Check sheet for the drawn part. Datum: minimum x, y, z corner. Units: mm. A direction names the side the tool comes from. Coordinates: 2 decimals unless noted, no trailing zeros. Write each loop counter-clockwise with the first axis right and the second up, starting at its lowest first coordinate (ties: lowest second). Pieces come first, ordered by that corner, then holes. Notation, with made-up numbers: M 76,31 L 108,31 A15 ccw 108,35 Z; hole C 86,13.5 d8. An arc over 180 degrees is marked long. Write item = value, one per line. Start each with the question number.
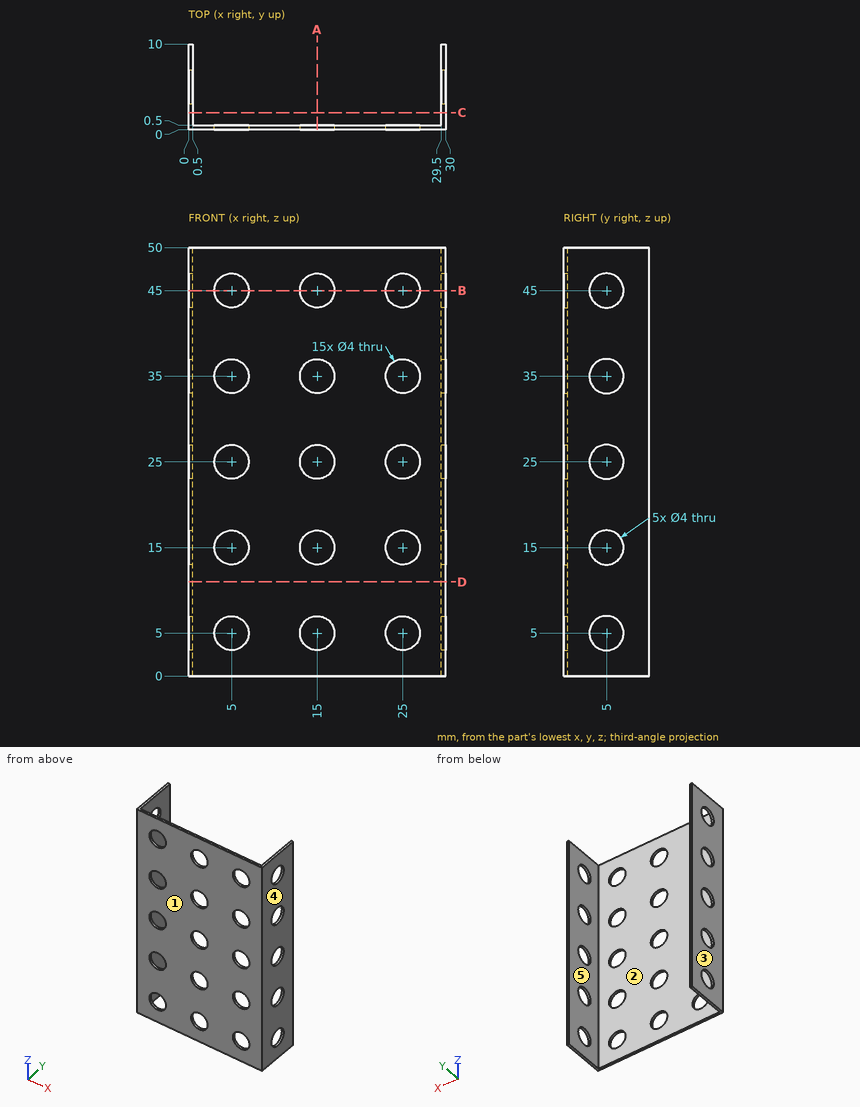
Q1. Cross-section at C-C on y = 2. Enter the section's corners in (x, z).
Q2. Cross-section at B-B on z = 45. Enter the section's corners in (x, y).
Q3. Scan lines: L1, parallel to Z at x = 25, y = 0.2; L2, parallel to X at y = 0.2, z = 35; L3, parallel to X at y = 8.5, z = 40.5. Record each from-to range of solid material in increasing order.
Q4. Gauge pin test, flat ends, axial feed: pin 1 (3.5 mm diameter, centred on y = 5, z = 15, fed in from +X); pin 2 (4.5 mm diameter, centred on x = 5, z = 15, fed in from +Y). Record the tip position at first contact, or that the pin passes through.
Q5. Draft check along X on the marked faces 1, 2 and 3. Enter one of: pulls with the +X half, pulls with the -X half, needs draft (parallel to the pull), parting line crosses it, or undercut.
Q6. Cross-section at A-A on x = 15. Enter the section's corners in (y, z).
Q7. Set-up check for the marked faces 4 and 5: record each of +Z, -Z, +X, -X, +Y, -Y from which the full face is reachable in a straight line by a thin tool's end or side.
Q8. Cross-section at D-D on z = 11. Enter the section's corners in (x, y), and give its area (3 significant figures).
Values found:
q1.outline = M 0,0 L 0.5,0 L 0.5,50 L 0,50 Z; M 29.5,0 L 30,0 L 30,50 L 29.5,50 Z
q2.outline = M 0,0 L 3,0 L 3,0.5 L 0.5,0.5 L 0.5,3 L 0,3 Z; M 0,7 L 0.5,7 L 0.5,10 L 0,10 Z; M 7,0 L 13,0 L 13,0.5 L 7,0.5 Z; M 17,0 L 23,0 L 23,0.5 L 17,0.5 Z; M 27,0 L 30,0 L 30,3 L 29.5,3 L 29.5,0.5 L 27,0.5 Z; M 29.5,7 L 30,7 L 30,10 L 29.5,10 Z
q3.L1 = 0 to 3, 7 to 13, 17 to 23, 27 to 33, 37 to 43, 47 to 50
q3.L2 = 0 to 3, 7 to 13, 17 to 23, 27 to 30
q3.L3 = 0 to 0.5, 29.5 to 30
q4.pin_1 = through
q4.pin_2 = 0.5
q5.face_1 = needs draft
q5.face_2 = undercut
q5.face_3 = pulls with the -X half
q6.outline = M 0,0 L 0.5,0 L 0.5,3 L 0,3 Z; M 0,7 L 0.5,7 L 0.5,13 L 0,13 Z; M 0,17 L 0.5,17 L 0.5,23 L 0,23 Z; M 0,27 L 0.5,27 L 0.5,33 L 0,33 Z; M 0,37 L 0.5,37 L 0.5,43 L 0,43 Z; M 0,47 L 0.5,47 L 0.5,50 L 0,50 Z
q7.face_4 = +Z, -Z, +X, +Y, -Y
q7.face_5 = +Z, -Z, +Y
q8.outline = M 0,0 L 30,0 L 30,10 L 29.5,10 L 29.5,0.5 L 0.5,0.5 L 0.5,10 L 0,10 Z
q8.area = 24.5 mm²
